Here's how the part is built. I have some questions about the finished solid (model axes, mm). Face numbers are marked on the shaded views. A direction names the side the tool comes from. Round coordinates to 2 decimals unless told otherwise and drop trailing zeros. Order: outer loops, then holes, each group sorted by start corner. A loop starts at its lowest first (then second) coordinate and runs counter-clockwise, first axis right, second up. Notation, with made-up numbers: M 39,34 L 50,34 A11 ccw 50,49 Z; hole C 86,9.25 d2. An arc over 180 degrees is marked long. Write item = value, one per line. Start each with the question number.
Item 1: I want a section at B-B, the plane y = 0. List the corners of the cut face in (x, z) for me.
Item 2: I want a section at A-A, the plane z = 14.5. List the corners of the cut face in (x, y) for me, plus the area to 3 significant figures.
Item 3: I'm going to push flat-ended pins straight in: P1, Ø6, axis at x = -8.5, y = 35.5, coming from the +Z side; P2, Ø5.5, axis at y = 26, z = 20.5, coming from the -X side; P3, Ø2, axis at x = 8.04, y = 0, coming from the +Z side; P4, Ø12, axis at x = 26, z = 13, coming from the -Y side. Where does each tip first touch, or does it pass through?
Item 4: Please list where these lines run through material, in increasing order: L1, parallel to X at y = -25, z = 5.5; L2, parallel to X at y = -25, z = 19.5; L3, parallel to Y at x = 33, z = 20.25.
Item 5: I want a section at C-C, the plane z = 5.75. State how many separate pieces and enclosed holes the cut face has, plus the area to 3 significant figures.
Item 6: I want a section at D-D, the plane x = -19.5. List the corners of the cut face in (y, z) for me, plus the area to 3 significant figures.
Item 7: For the marked faces 1 and 2, which set-ups out of +Z, -Z, +X, -X, +Y, -Y let a thin tool reach every point of the face, with its end or its side?
```python
from build123d import *

# Parameters (mm, degrees)
SKETCH1_W           = 40
SKETCH1_H           = 130.000000968
SKETCH1_R           = 2.25
SKETCH1_R_2         = 1.4
BOSS_EXTRUDE1_DEPTH = 10
SKETCH1_3_R         = 1.4
BOSS_EXTRUDE2_DEPTH = 28.45


with BuildPart() as part:
    # Sketch1 → Boss-Extrude1 (new body)
    with BuildSketch(Plane.XY):
        with Locations((-23.042, 0)):
            Rectangle(SKETCH1_W, SKETCH1_H)
        with Locations((-10.042, 55.000000484)):
            Circle(SKETCH1_R, mode=Mode.SUBTRACT)
        with Locations((-36.042, -54.999999516)):
            Circle(SKETCH1_R, mode=Mode.SUBTRACT)
        with Locations((-10.042, -54.999999516)):
            Circle(SKETCH1_R, mode=Mode.SUBTRACT)
        with Locations((-36.042, 55.000000484)):
            Circle(SKETCH1_R, mode=Mode.SUBTRACT)
        with BuildLine():
            Line((43.042, -25.000000484), (43.042, 25.000000484))
            ThreePointArc((43.042, 25.000000484), (31.326271247, 53.284271732), (3.042, 65.000000484))
            Line((3.042, 65.000000484), (-3.042, 65.000000484))
            Line((-3.042, 65.000000484), (-3.042, -65.000000484))
            Line((-3.042, -65.000000484), (3.042, -65.000000484))
            ThreePointArc((3.042, -65.000000484), (31.326271247, -53.284271732), (43.042, -25.000000484))
        make_face()
        with Locations((32.041768895, 0)):
            Circle(SKETCH1_R_2, mode=Mode.SUBTRACT)
        with Locations((32.041768895, -25.000000484)):
            Circle(SKETCH1_R_2, mode=Mode.SUBTRACT)
        with Locations((32.041768895, 25.000000484)):
            Circle(SKETCH1_R_2, mode=Mode.SUBTRACT)
        with Locations((8.041768895, 0)):
            Circle(SKETCH1_R_2, mode=Mode.SUBTRACT)
        with Locations((8.041768895, 25.000000484)):
            Circle(SKETCH1_R_2, mode=Mode.SUBTRACT)
        with Locations((8.041768895, -25.000000484)):
            Circle(SKETCH1_R_2, mode=Mode.SUBTRACT)
    extrude(amount=BOSS_EXTRUDE1_DEPTH)

    # Sketch1_3 → Boss-Extrude2 (add)
    with BuildSketch(Plane.XY):
        with BuildLine():
            Line((43.042, -25.000000484), (43.042, 25.000000484))
            ThreePointArc((43.042, 25.000000484), (31.326271247, 53.284271732), (3.042, 65.000000484))
            Line((3.042, 65.000000484), (-3.042, 65.000000484))
            Line((-3.042, 65.000000484), (-3.042, -65.000000484))
            Line((-3.042, -65.000000484), (3.042, -65.000000484))
            ThreePointArc((3.042, -65.000000484), (31.326271247, -53.284271732), (43.042, -25.000000484))
        make_face()
        with Locations((32.041768895, 0)):
            Circle(SKETCH1_3_R, mode=Mode.SUBTRACT)
        with Locations((32.041768895, -25.000000484)):
            Circle(SKETCH1_3_R, mode=Mode.SUBTRACT)
        with Locations((32.041768895, 25.000000484)):
            Circle(SKETCH1_3_R, mode=Mode.SUBTRACT)
        with Locations((8.041768895, 0)):
            Circle(SKETCH1_3_R, mode=Mode.SUBTRACT)
        with Locations((8.041768895, 25.000000484)):
            Circle(SKETCH1_3_R, mode=Mode.SUBTRACT)
        with Locations((8.041768895, -25.000000484)):
            Circle(SKETCH1_3_R, mode=Mode.SUBTRACT)
    extrude(amount=BOSS_EXTRUDE2_DEPTH)


solid = part.part
```
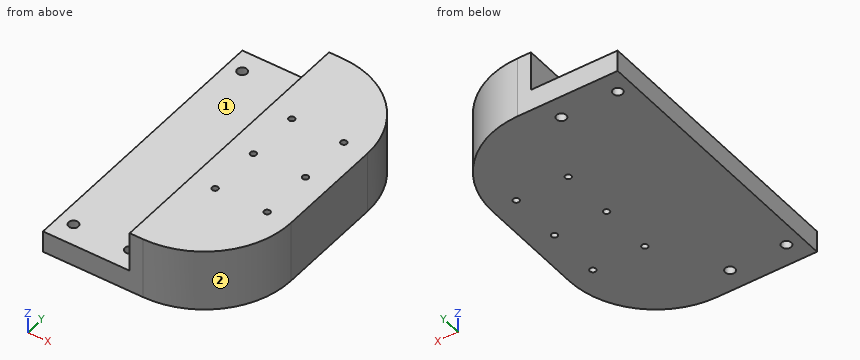
Filled in:
q1.outline = M -43.04,0 L 6.64,0 L 6.64,28.45 L -3.04,28.45 L -3.04,10 L -43.04,10 Z; M 9.44,0 L 30.64,0 L 30.64,28.45 L 9.44,28.45 Z; M 33.44,0 L 43.04,0 L 43.04,28.45 L 33.44,28.45 Z
q2.outline = M -3.04,-65 L 3.04,-65 A40 ccw 43.04,-25 L 43.04,25 A40 ccw 3.04,65 L -3.04,65 Z; hole C 8.04,-25 d2.8; hole C 8.04,0 d2.8; hole C 8.04,25 d2.8; hole C 32.04,-25 d2.8; hole C 32.04,0 d2.8; hole C 32.04,25 d2.8
q2.area = 5,270 mm^2
q3.P1 = 10
q3.P2 = -3.04
q3.P3 = through
q3.P4 = -61.23
q4.L1 = -43.04 to 6.64, 9.44 to 30.64, 33.44 to 43.04
q4.L2 = -3.04 to 6.64, 9.44 to 30.64, 33.44 to 43.04
q4.L3 = -51.51 to -26.02, -23.98 to -1.02, 1.02 to 23.98, 26.02 to 51.51
q5.separate_pieces = 1
q5.enclosed_holes = 10
q5.area = 10,400 mm^2
q6.outline = M -65,0 L 65,0 L 65,10 L -65,10 Z
q6.area = 1,300 mm^2
q7.face_1 = +Z, -X, +Y, -Y
q7.face_2 = +Z, -Z, +X, -Y
